Source: CAD feature listing. Evaluate the final solid. Frame: model axes, mm. A direction names the side the tool comes from. Round coordinates to 2 decimals unless told otherwise and drop trailing zeros. Loops run counter-clockwise (first coordinate to the right, second up) from the corner with the lowest first, then second, coordinate; pieces in that order, holes last.
Item 1: First-contact query: P1, Ø1, axis at x = 20, y = 2, coming from the +Z side; P2, Ø0.9, axis at x = -15.5, z = 2, coming from the +Y side; P3, Ø1.5, axis at x = -7.5, z = 3, coming from the -Y side; P4, Ø4, axis at x = -2, y = 0.5, coming from the +Z side. Flat tips, straight axial feed; report the tip coordinate or a pass-through.
Item 2: Access query for faces 1 (the flat face through (-59, -7, 0.6)), 2 (the flat face through (44, -2, 2)), 3 (the cylindrical face through (19, 3, 3)), 4 (the cylindrical face through (17, 3, 2)), 5 (the flat face through (45, 2, 2)). Directions: +Z, -Z, +X, -X, +Y, -Y. A direction counts if a zero-diameter tool reaches every point of the face in a straight line with its end or side. Return the directions, or none.
Item 3: Pull-direction query (Y, two-part tool) for faces 6 (the cylindrical face through (23, 3, 3)), 7 (the cylindrical face through (-55, -3, 2)), 8 (the flat face through (-19.2, -1.8, 4)); classes: released by +Y, released by -Y, zero draft, split by the parting line, or undercut.
Item 4: Ray query, L1, parallel to Y at x = -41.5, z = 2.65; L2, parallel to X at y = -4, z = 1.7; L3, parallel to X at y = -6, z = 1.85. Return the intervals inside material, ascending.
Item 5: Section query B-B on z = 1.7. Give the number of separate pieces and of enclosed holes in the cut face, then the cut area to 3 significant figures.
Item 6: Section query C-C on x = -50. Return loops of the section in (y, z).
Item 7: Section query A-A on y = -3. Return loops of the section in (x, z).
```python
from build123d import *

# Parameters (mm, degrees)
F0_W     = 4
F0_H     = 5
F0_W_2   = 76
F0_H_2   = 2
F1_DEPTH = 1
F2_W     = 1
F2_H     = 14
F2_W_2   = 6
F2_H_2   = 1
F2_W_3   = 5
F2_W_4   = 33
F2_W_5   = 65
F3_DEPTH = 3
F4_R     = 4.99999
F5_R     = 4.99999


# Not quite as in the source:
# - a fillet or chamfer is up to 0.001 mm smaller than in the source, because OpenCascade refuses the exact size


with BuildPart() as f1:
    # F0 (on Top) → F1 (new body)
    with BuildSketch(Plane.XY):
        with Locations((-59, 4.5)):
            Rectangle(F0_W, F0_H)
        with Locations((-19, -1)):
            Rectangle(F0_W_2, F0_H_2)
        with Locations((-19, 1)):
            Rectangle(F0_W_2, F0_H_2)
        with Locations((-59, -1)):
            Rectangle(F0_W, F0_H_2)
        with Locations((-59, 1)):
            Rectangle(F0_W, F0_H_2)
        with Locations((-59, -4.5)):
            Rectangle(F0_W, F0_H)
        Polygon((61, 2), (23, 2), (23, 0), (23, -2), (61, -2), align=None)
        with Locations((21, 1)):
            Rectangle(F0_W, F0_H_2)
        with Locations((21, -1)):
            Rectangle(F0_W, F0_H_2)
        with Locations((21, 4.5)):
            Rectangle(F0_W, F0_H)
        with Locations((21, -4.5)):
            Rectangle(F0_W, F0_H)
    extrude(amount=F1_DEPTH)

    # F2 (on face) → F3 (join)
    with BuildSketch(Plane.XY.offset(1)):
        with Locations((-60.5, 0)):
            Rectangle(F2_W, F2_H)
        Polygon((-57, 7), (-58, 7), (-58, 1), (-57, 1), (-57, 2), align=None)
        with Locations((-54, 1.5)):
            Rectangle(F2_W_2, F2_H_2)
        with Locations((-54, -1.5)):
            Rectangle(F2_W_2, F2_H_2)
        Polygon((-58, -1), (-58, -7), (-57, -7), (-57, -2), (-57, -1), align=None)
        Polygon((19, -1), (19, -2), (19, -7), (20, -7), (20, -1), align=None)
        Polygon((19, 7), (19, 2), (19, 1), (20, 1), (20, 7), align=None)
        with Locations((16.5, 1.5)):
            Rectangle(F2_W_3, F2_H_2)
        with Locations((16.5, -1.5)):
            Rectangle(F2_W_3, F2_H_2)
        with Locations((25.5, -1.5)):
            Rectangle(F2_W_3, F2_H_2)
        with Locations((25.5, 1.5)):
            Rectangle(F2_W_3, F2_H_2)
        Polygon((23, 7), (22, 7), (22, 1), (23, 1), (23, 2), align=None)
        Polygon((22, -1), (22, -7), (23, -7), (23, -2), (23, -1), align=None)
        with Locations((44.5, -1.5)):
            Rectangle(F2_W_4, F2_H_2)
        with Locations((-18.5, 1.5)):
            Rectangle(F2_W_5, F2_H_2)
        with Locations((-18.5, -1.5)):
            Rectangle(F2_W_5, F2_H_2)
        with Locations((44.5, 1.5)):
            Rectangle(F2_W_4, F2_H_2)
    extrude(amount=F3_DEPTH)

    # F4 (radius 5 in the source; OpenCascade refuses exactly that, so slightly less here)
    f4_edges = [f1.edges().sort_by_distance(p)[0] for p in [
        (23, -2, 2),
        (20, -1, 2.5),
        (20, 1, 2.5),
        (22, 1, 2.5),
        (19, -2, 2),
        (22, -1, 2.5),
        (19, 2, 2),
        (23, 2, 2),
    ]]
    fillet(f4_edges, radius=F4_R)

    # F5 (radius 5 in the source; OpenCascade refuses exactly that, so slightly less here)
    f5_edges = [f1.edges().sort_by_distance(p)[0] for p in [
        (-57, -2, 2),
        (-58, 1, 2.5),
        (-57, 2, 2),
        (-58, -1, 2.5),
    ]]
    fillet(f5_edges, radius=F5_R)


solid = f1.part
```
Data:
1. P1: stops at z = 1
1. P2: stops at y = 2
1. P3: stops at y = -2
1. P4: stops at z = 4
2. face 1: +Z, -Z, +X, -X, -Y
2. face 2: +Z, -Z, +X, -Y
2. face 3: +Z
2. face 4: +Z, -Z, +Y
2. face 5: +Z, -Z, +X, +Y
3. face 6: undercut
3. face 7: released by -Y
3. face 8: zero draft
4. L1: y = -2 to -1, 1 to 2
4. L2: x = -61 to -60, -57.58 to -56, 18 to 19.58, 22.42 to 24
4. L3: x = -61 to -60, -58 to -56.9, 18.9 to 20, 22 to 23.1
5. separate pieces: 5
5. enclosed holes: 0
5. area: 278 mm2
6. outline: (-2, 0) - (2, 0) - (2, 4) - (1, 4) - (1, 1) - (-1, 1) - (-1, 4) - (-2, 4) - close
7. outline: (-61, 0) - (-55, 0) - (-55, 4) - (-57, 4) - (-57, 1) - (-60, 1) - (-60, 4) - (-61, 4) - close; (17, 0) - (25, 0) - (25, 4) - (23, 4) - (23, 1) - (19, 1) - (19, 4) - (17, 4) - close
